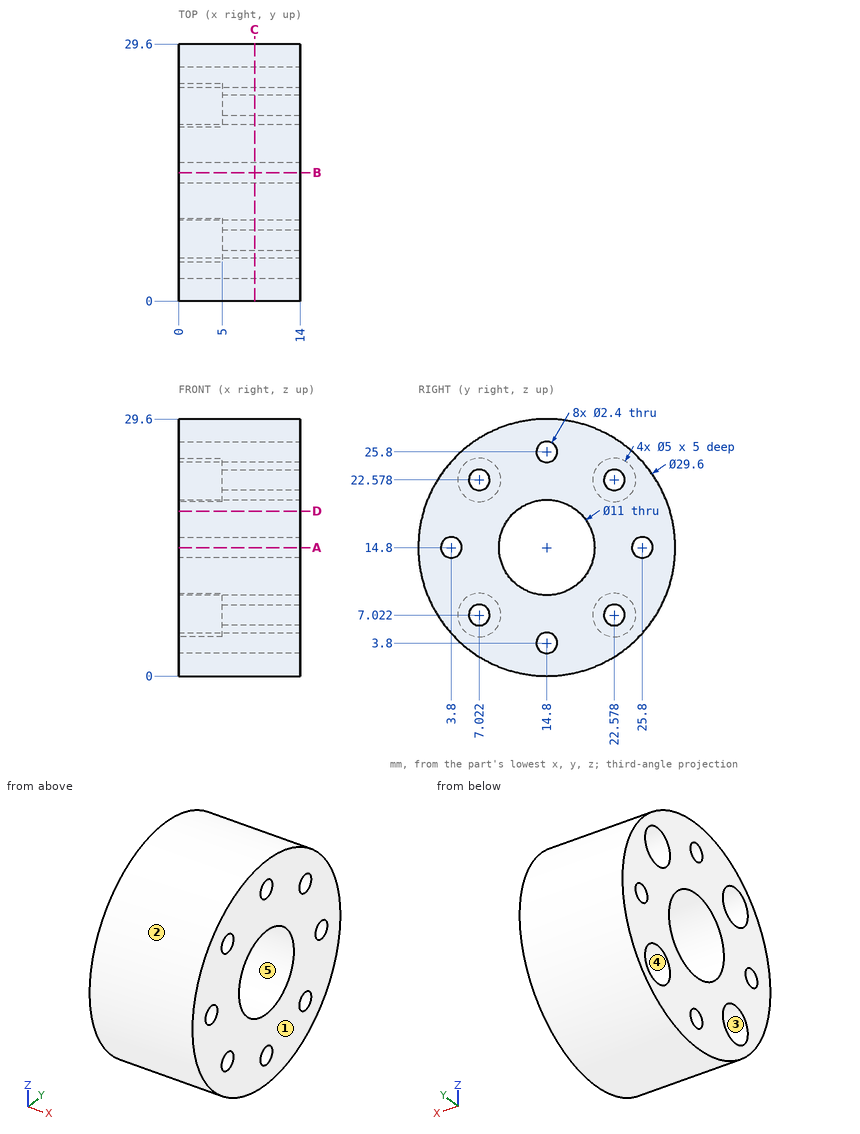
Job drawing, mm, ordinate dimensions from the low corner. One solid piece. A direction names the side the tool comes from. Coordinates: 2 decimals unless noted, no trailing zeros. Write each loop counter-clockwise with the first axis right and the second up, starting at its lowest first coordinate (ties: lowest second). Pieces come first, ordered by that corner, then holes. Notation, with made-up numbers: (35, 52.25) -> (87, 52.25) arc R24 ccw to (87, 65.25) -> close; hole circle Ø9 at (-10, -12.75). An arc over 180 degrees is marked (long way). Use CSV: the item, a comma, the result in double quotes. Start each with the question number.
Item 1: Tool access for the marked faces 4 and 5: list every direction of +Z, -Z, +X, -X, +Y, -Y with a clear straight run to the whole face (end or side of a thin tool).
Item 2: Two-plate mould, pull along Z, no slides. Class the marked faces 1, 2 and 3: +Z half, -Z half, draft (parallel to the pull), parting line (faces both ways), or undercut.
Item 3: Band-saw the part on C-C, the plane x = 8.75. Give the number of separate pieces and of enclosed holes in the cut face, plus the area to 3 significant figures.
Item 4: Drop flat-ended pins along their axis: P1, Ø2, axis at x = 7, z = 9.5, coming from the +Y side; P2, Ø1.4, axis at y = 14.8, z = 3.8, coming from the -X side; P3, Ø6, axis at x = 10, y = 21.5, coming from the +Z side; P4, Ø4, axis at x = 7.5, z = 19.5, coming from the -Y side. Give the stop position or say it passes through.
Item 5: Band-saw the part on A-A, the plane z = 14.8. Write the cut outline in (x, y), plus the area to 3 significant figures.
Item 6: Wall check: probe 1 along Y at (x, z) = (5.25, 14.75); probe 2 along Z at (x, y) = (9.75, 23.25); probe 3 along Y at (x, z) = (13.5, 6.5). Give the ranges that are in metal, low to high.
Item 7: Band-saw the part on D-D, the plane z = 19. Write the cut outline in (x, y), plus the area to 3 significant figures.
Response values:
1,face 4,"-X"
1,face 5,"+X, -X"
2,face 1,"draft"
2,face 2,"parting line"
2,face 3,"undercut"
3,separate pieces,"1"
3,enclosed holes,"9"
3,area,"557 mm2"
4,P1,"stops at y = 28.96"
4,P2,"passes through"
4,P3,"stops at z = 29.13"
4,P4,"stops at y = 0.25"
5,outline,"(0, 0) -> (14, 0) -> (14, 2.6) -> (0, 2.6) -> close; (0, 5) -> (14, 5) -> (14, 9.3) -> (0, 9.3) -> close; (0, 20.3) -> (14, 20.3) -> (14, 24.6) -> (0, 24.6) -> close; (0, 27) -> (14, 27) -> (14, 29.6) -> (0, 29.6) -> close"
5,area,"193 mm2"
6,probe 1,"y = 0 to 2.6, 5 to 9.3, 20.3 to 24.6, 27 to 29.6"
6,probe 2,"z = 2.65 to 6.03, 8.02 to 21.58, 23.57 to 26.95"
6,probe 3,"y = 2.55 to 5.94, 8.1 to 21.5, 23.66 to 27.05"
7,outline,"(0, 0.61) -> (14, 0.61) -> (14, 11.25) -> (0, 11.25) -> close; (0, 18.35) -> (14, 18.35) -> (14, 28.99) -> (0, 28.99) -> close"
7,area,"298 mm2"
